```python
from build123d import *

# Parameters (mm, degrees)
SKETCH_1_W          = 35.6
SKETCH_1_H          = 50.6
EXTRUDE_1_DEPTH     = 1.5
SKETCH_2_W          = 23.7
SKETCH_2_H          = 4.8
SKETCH_2_R          = 1.5
EXTRUDE_2_DEPTH     = 2
SKETCH_2_3_R        = 2.25
CUT_EXTRUDE_1_DEPTH = 1
SKETCH_3_W          = 2.8
SKETCH_3_H          = 1.3
EXTRUDE_3_DEPTH     = 2
FILLET_1_R          = 5


with BuildPart() as part:
    # 草图1 → 凸台-拉伸1 (new body)
    with BuildSketch(Plane(origin=(0, 0, 0), x_dir=(1, 0, 0), z_dir=(0, 1, 0))):
        with Locations((17.8, -25.3)):
            Rectangle(SKETCH_1_W, SKETCH_1_H)
    extrude(amount=EXTRUDE_1_DEPTH)

    # 草图2 → 凸台-拉伸2 (add)
    with BuildSketch(Plane.XZ):
        with Locations((23.75, 53)):
            Rectangle(SKETCH_2_W, SKETCH_2_H)
        with Locations(Location((23.8, 52.8, 0), (0, 0, 270))):
            Circle(SKETCH_2_R, mode=Mode.SUBTRACT)
    extrude(amount=-EXTRUDE_2_DEPTH)

    # 草图2<3> → 切除-拉伸1 (cut)
    with BuildSketch(Plane.XZ):
        with Locations(Location((23.8, 52.8, 0), (0, 0, 270))):
            Circle(SKETCH_2_3_R)
    extrude(amount=-CUT_EXTRUDE_1_DEPTH, mode=Mode.SUBTRACT)

    # 草图3 → 凸台-拉伸3 (add)
    with BuildSketch(Plane(origin=(0, 0, 0), x_dir=(-1, 0, 0), z_dir=(0, 0, -1))):
        with Locations((-23.8, 1.75)):
            Rectangle(SKETCH_3_W, SKETCH_3_H)
        with Locations((-11.8, 1.75)):
            Rectangle(SKETCH_3_W, SKETCH_3_H)
    extrude(amount=EXTRUDE_3_DEPTH)

    # 圆角1
    # the kernel refuses this fillet: 5 mm, written as the material it adds along each edge
    with BuildSketch(Plane(origin=(13.2, 1.5, 0), x_dir=(0, 0, 1), z_dir=(-1, 0, 0)), Plane(origin=(25.2, 1.5, 0), x_dir=(0, 0, 1), z_dir=(-1, 0, 0))) as fillet_1_piece_1:
        with BuildLine():
            CenterArc((2.861817604, 5), FILLET_1_R, 235.084793753, 34.915206247)
            Line((0, 0.9), (0, 0))
            Line((0, 0), (2.861817604, 0))
        make_face()
    extrude(amount=2.8)


solid = part.part
```
For this review, take the finished solid that the model builds, in its own axes (mm). A direction names the side the tool comes from. Give positions to 0.01 mm unless a question says otherwise; leave off trailing zeros. Write each loop counter-clockwise with the first axis right and the second up, starting at its lowest first coordinate (ties: lowest second). Pieces come first, ordered by that corner, then holes. Notation, with made-up numbers: M -29,-28.5 L 4,-28.5 A22 cw 4,-3.5 Z; hole C 12,-31 d5. An arc over 180 degrees is marked long. Answer as CSV lines item,"result".
1. Consider section C-C, the plane y = 0.45. Write out the cut boundary in (x, z).
Findings:
outline,"M 0,0 L 35.6,0 L 35.6,55.4 L 11.9,55.4 L 11.9,50.6 L 0,50.6 Z; hole C 23.8,52.8 d4.5"
2. Consider section A-A, the plane z = 52.8. Write out the cut boundary in (x, y).
Findings:
outline,"M 11.9,0 L 21.55,0 L 21.55,1 L 22.3,1 L 22.3,2 L 11.9,2 Z; M 25.3,1 L 26.05,1 L 26.05,0 L 35.6,0 L 35.6,2 L 25.3,2 Z"
3. For faces 1 (the cylindrical face through (11.82, 1.737, 1.341)), 2 (the flat face through (6, 1, 50.6)), 3 (the flat face through (24, 2, 55)), list the 3-axis set-ups (+Z, -Z, +X, -X, +Y, -Y) from which the entire face can be reached by the end or side of a thin tool; tool diameter is ignored.
Findings:
face 1,"+X, -X, +Y"
face 2,"+Z, -X, +Y, -Y"
face 3,"+Z, +X, -X, +Y"
4. Draft analysis for pull direction X (two halves, no side actions). For faces 4 (the flat face through (22.4, 2, -1)), 5 (the flat face through (24, 1, 55.4)), 6 (the flat face through (11.9, 1, 53)), state which applies: +X half, -X half, draft (parallel to the pull), parting line (faces both ways), or undercut.
Findings:
face 4,"undercut"
face 5,"draft"
face 6,"-X half"
5. Consider section B-B, the plane x = 23.8. Write out the cut boundary in (y, z), then the cut area to 3 significant figures.
Findings:
outline,"M 0,0 L 1.1,0 L 1.1,-2 L 2.4,-2 L 2.4,0 A5 cw 1.5,2.86 L 1.5,50.6 L 2,50.6 L 2,51.3 L 1,51.3 L 1,50.55 L 0,50.55 Z; M 0,55.05 L 1,55.05 L 1,54.3 L 2,54.3 L 2,55.4 L 0,55.4 Z"
area,"81.4 mm2"
6. Wall thickness on line 1 (X direction, y = 1.55, z = 52.8); line 2 (Y direction, x = 11.5, z = 20); line 3 (Y direction, x = 12.5, z = 53.5): over which ranges is each line inside the solid? List them lowest first.
Findings:
line 1,"x = 11.9 to 22.3, 25.3 to 35.6"
line 2,"y = 0 to 1.5"
line 3,"y = 0 to 2"
7. Consider section D-D, the plane x = 17. Write out the cut boundary in (y, z).
Findings:
outline,"M 0,0 L 1.5,0 L 1.5,50.6 L 2,50.6 L 2,55.4 L 0,55.4 Z"
8. For pin 1 (3 mm diameter, centred on x = 19.5, z = 44, fed in from +Y); pin 2 (1 mm diameter, centred on y = 1, z = 54, fed in from -X); pin 3 (1.2 mm diameter, centred on x = 7, y = 1, fed in from +Z), all flat-tipped, find the tip position at first contact; note any pin that passes through.
Findings:
pin 1,"stops at y = 1.5"
pin 2,"stops at x = 11.9"
pin 3,"stops at z = 50.6"
